```python
from build123d import *

# Parameters (mm, degrees)
F1_DEPTH  = 6.35
F2_W      = 7.9056663411
F2_H      = 7.9056663411
F3_DEPTH  = 25.4
F4_W      = 6.858
F4_H      = 6.858
F5_DEPTH  = 25.4
F6_W      = 7.9056663411
F6_H      = 8.1499283314
F6_W_2    = 8.1499283314
F6_H_2    = 7.9056663411
F7_DEPTH  = 1.27
F8_SIZE   = 1.26999
F10_DEPTH = 6.35


# Not quite as in the source:
# - a fillet or chamfer is up to 0.001 mm smaller than in the source, because OpenCascade refuses the exact size
# - a feature names something its author has since deleted; it is built from what else it names


with BuildPart() as f1:
    # F0 (on Top) → F1 (new body)
    with BuildSketch(Plane.XY):
        with BuildLine():
            ThreePointArc((13.6716806904, 59.1812469065), (-3.4947036843, 66.2917961397), (3.6158455206, 49.1254117533))
            ThreePointArc((3.6158455206, 49.1254117533), (10.7263947587, 52.0706976733), (13.6716806904, 59.1812469065))
        make_face()
    extrude(amount=F1_DEPTH)

    # F4 (on face) → F5 (cut)
    with BuildSketch(Plane.XY.offset(6.35)):
        with Locations((3.6158455372, 59.1812469065)):
            Rectangle(F4_W, F4_H)
    extrude(amount=-F5_DEPTH, mode=Mode.SUBTRACT)



with BuildPart() as f1b:
    # F0 (on Top) → F1, piece 2 (new body)
    with BuildSketch(Plane.XY):
        Polygon((3.6158455206, 49.1254117533), (-34.4841544628, 49.1254117533), (-34.4841544628, -27.0745882467), (41.7158455372, -27.0745882467), (41.7158455372, 49.1254117533), align=None)
    extrude(amount=F1_DEPTH)

    # F2 (on face) → F3 (cut)
    with BuildSketch(Plane.XY.offset(6.35)):
        Polygon((-34.4841544628, 33.0698170808), (-26.3342261314, 33.0698170808), (-18.4285597903, 33.0698170808), (-18.4285597903, 40.9754834219), (-18.4285597903, 49.1254117533), (-34.4841544628, 49.1254117533), align=None)
        Polygon((25.6602508647, 40.9754834219), (25.6602508647, 33.0698170808), (33.5659172058, 33.0698170808), (41.7158455372, 33.0698170808), (41.7158455372, 49.1254117533), (25.6602508647, 49.1254117533), align=None)
        Polygon((33.5659172058, -11.0189935742), (25.6602508647, -11.0189935742), (25.6602508647, -18.9246599153), (25.6602508647, -27.0745882467), (41.7158455372, -27.0745882467), (41.7158455372, -11.0189935742), align=None)
        Polygon((-18.4285597903, -18.9246599153), (-18.4285597903, -11.0189935742), (-26.3342261314, -11.0189935742), (-34.4841544628, -11.0189935742), (-34.4841544628, -27.0745882467), (-18.4285597903, -27.0745882467), align=None)
        with Locations((-22.3813929609, 1.0837679277)):
            Rectangle(F2_W, F2_H)
        with Locations((-22.3813929609, 20.9670555789)):
            Rectangle(F2_W, F2_H)
        with Locations((-6.3257982884, 37.0226502514)):
            Rectangle(F2_W, F2_H)
        with Locations((-6.3257982884, 20.9670555789)):
            Rectangle(F2_W, F2_H)
        with Locations((-6.3257982884, 1.0837679277)):
            Rectangle(F2_W, F2_H)
        with Locations((-6.3257982884, -14.9718267448)):
            Rectangle(F2_W, F2_H)
        with Locations((13.5574893628, -14.9718267448)):
            Rectangle(F2_W, F2_H)
        with Locations((13.5574893628, 1.0837679277)):
            Rectangle(F2_W, F2_H)
        with Locations((29.6130840353, 1.0837679277)):
            Rectangle(F2_W, F2_H)
        with Locations((29.6130840353, 20.9670555789)):
            Rectangle(F2_W, F2_H)
        with Locations((13.5574893628, 20.9670555789)):
            Rectangle(F2_W, F2_H)
        with Locations((13.5574893628, 37.0226502514)):
            Rectangle(F2_W, F2_H)
    extrude(amount=-F3_DEPTH, mode=Mode.SUBTRACT)

    # F6 (on face) → F7 (join, symmetric)
    with BuildSketch(Plane.XY.offset(6.35)):
        with Locations((-22.3813929609, 28.9948529151)):
            Rectangle(F6_W, F6_H)
        with Locations((-14.3535956246, 28.9948529151)):
            Rectangle(F6_W_2, F6_H)
        with Locations((-14.3535956246, 37.0226502514)):
            Rectangle(F6_W_2, F6_H_2)
        with Locations((-6.3257982884, 28.9948529151)):
            Rectangle(F6_W, F6_H)
        with Locations((-14.3535956246, 20.9670555789)):
            Rectangle(F6_W_2, F6_H_2)
        with Locations((13.5574893628, 28.9948529151)):
            Rectangle(F6_W, F6_H)
        with Locations((29.6130840353, 28.9948529151)):
            Rectangle(F6_W, F6_H)
        with Locations((21.585286699, 28.9948529151)):
            Rectangle(F6_W_2, F6_H)
        with Locations((21.585286699, 37.0226502514)):
            Rectangle(F6_W_2, F6_H_2)
        with Locations((21.585286699, 20.9670555789)):
            Rectangle(F6_W_2, F6_H_2)
        with Locations((-14.3535956246, 1.0837679277)):
            Rectangle(F6_W_2, F6_H_2)
        with Locations((-14.3535956246, -6.9440294085)):
            Rectangle(F6_W_2, F6_H)
        with Locations((-14.3535956246, -14.9718267448)):
            Rectangle(F6_W_2, F6_H_2)
        with Locations((-22.3813929609, -6.9440294085)):
            Rectangle(F6_W, F6_H)
        with Locations((-6.3257982884, -6.9440294085)):
            Rectangle(F6_W, F6_H)
        with Locations((13.5574893628, -6.9440294085)):
            Rectangle(F6_W, F6_H)
        with Locations((21.585286699, -6.9440294085)):
            Rectangle(F6_W_2, F6_H)
        with Locations((29.6130840353, -6.9440294085)):
            Rectangle(F6_W, F6_H)
        with Locations((21.585286699, -14.9718267448)):
            Rectangle(F6_W_2, F6_H_2)
        with Locations((21.585286699, 1.0837679277)):
            Rectangle(F6_W_2, F6_H_2)
    extrude(amount=F7_DEPTH, both=True)

    # F8 (size 1.27 in the source; OpenCascade refuses exactly that, so slightly less here)
    f8_edges = [f1b.edges().sort_by_distance(p)[0] for p in [
        (-22.381393, 33.069817, 7.62),
        (-18.42856, 37.02265, 7.62),
        (-14.353596, 40.975483, 7.62),
        (-10.278631, 37.02265, 7.62),
        (-6.325798, 33.069817, 7.62),
        (-2.372965, 28.994853, 7.62),
        (-6.325798, 24.919889, 7.62),
        (-10.278631, 20.967056, 7.62),
        (-14.353596, 17.014222, 7.62),
        (-18.42856, 20.967056, 7.62),
        (-22.381393, 24.919889, 7.62),
        (-26.334226, 28.994853, 7.62),
        (-10.278631, 1.083768, 7.62),
        (-6.325798, -2.869065, 7.62),
        (-2.372965, -6.944029, 7.62),
        (-6.325798, -11.018994, 7.62),
        (-14.353596, -18.92466, 7.62),
        (-26.334226, -6.944029, 7.62),
        (-22.381393, -11.018994, 7.62),
        (-18.42856, -14.971827, 7.62),
        (-22.381393, -2.869065, 7.62),
        (-18.42856, 1.083768, 7.62),
        (-14.353596, 5.036601, 7.62),
        (-10.278631, -14.971827, 7.62),
        (25.660251, 1.083768, 7.62),
        (25.660251, -14.971827, 7.62),
        (21.585287, -18.92466, 7.62),
        (17.510323, -14.971827, 7.62),
        (13.557489, -11.018994, 7.62),
        (9.604656, -6.944029, 7.62),
        (13.557489, -2.869065, 7.62),
        (17.510323, 1.083768, 7.62),
        (21.585287, 5.036601, 7.62),
        (29.613084, -2.869065, 7.62),
        (29.613084, -11.018994, 7.62),
        (33.565917, -6.944029, 7.62),
        (29.613084, 33.069817, 7.62),
        (25.660251, 37.02265, 7.62),
        (21.585287, 40.975483, 7.62),
        (17.510323, 37.02265, 7.62),
        (13.557489, 33.069817, 7.62),
        (9.604656, 28.994853, 7.62),
        (17.510323, 20.967056, 7.62),
        (13.557489, 24.919889, 7.62),
        (21.585287, 17.014222, 7.62),
        (29.613084, 24.919889, 7.62),
        (33.565917, 28.994853, 7.62),
        (25.660251, 20.967056, 7.62),
    ]]
    chamfer(f8_edges, length=F8_SIZE)


with BuildPart() as f1_1:
    add(f1.part)

    add(f1b.part)  # F10 merges F1b
    # F9 (on face) → F10 (join)
    with BuildSketch(Plane.XY.offset(6.35)):
        with BuildLine():
            Line((-6.439989616, 49.1254117533), (3.6158455372, 49.1254117533))
            ThreePointArc((3.6158455372, 49.1254117533), (-3.4947036902, 52.0706976792), (-6.439989616, 59.1812469065))
            Line((-6.439989616, 59.1812469065), (-6.439989616, 49.1254117533))
        make_face()
        with BuildLine():
            Line((3.6158455372, 49.1254117533), (13.6716806904, 49.1254117533))
            Line((13.6716806904, 49.1254117533), (13.6716806904, 59.1812469065))
            ThreePointArc((13.6716806904, 59.1812469065), (10.7263947645, 52.0706976792), (3.6158455372, 49.1254117533))
        make_face()
    extrude(amount=-F10_DEPTH)


solid = f1_1.part
```
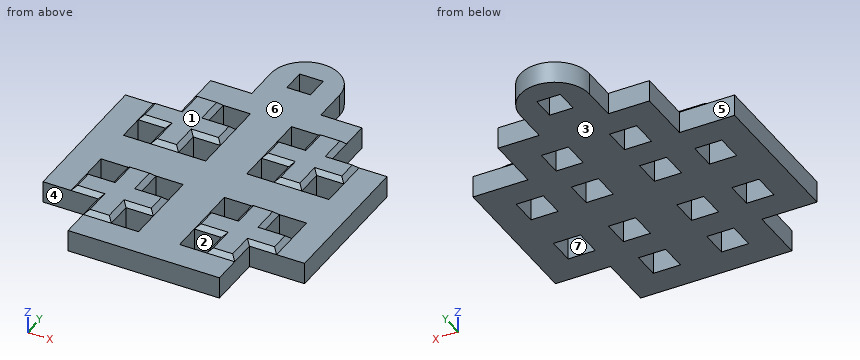
For this review, take the finished solid that the model builds, in its own axes (mm). Face numbers are marked on the shaded views. A direction names the side the tool comes from. Coordinates: 2 decimals unless noted, no trailing zeros. Order: outer loops, then holes, each group sorted by start corner. A loop starts at its lowest first (then second) coordinate and runs counter-clockwise, first axis right, second up. Notation, with made-up numbers: (29.5, 58) -> (74.5, 58) arc R17 ccw to (74.5, 89) -> close; hole circle Ø6 at (66.25, -37.5). An arc over 180 degrees is marked (long way). Use CSV: the item, a comma, the result in double quotes. Start each with the question number.
Item 1: Draft analysis for pull direction X (two halves, no side actions). For the marked faces 1 and 2, state which applies: pulls with the +X half, pulls with the -X half, needs draft (parallel to the pull), parting line crosses it, or undercut.
Item 2: Wall thickness on probe 1 along X at (y, z) = (3, 3.75); probe 2 along Y at (x, z) = (-21.5, 4.5); probe 3 along Y at (x, z) = (-30.5, 6): over which ranges is each line inside the solid? List them lowest first.
Item 3: We need section B-B, the plane y = 1.5. Give the boundary of the cut face in (x, z).
Item 4: We need section A-A, the plane x = 29. Give the boundary of the cut face in (y, z).
Item 5: Insertion check: pin 1 (3 mm diameter, centred on x = -22.5, z = 4, fed in from +Y); pin 2 (1.5 mm diameter, centred on x = -1.5, z = 5, fed in from +Y); pin 3 (3 mm diameter, centred on y = -14.5, z = 2.5, fed in from -X). Each pin has a flat end and moves straight along its axis. Give the tip position at first contact, or say it passes through.
Item 6: For the marked faces 3, 4, 5, 6 and 7, list the 3-axis set-ups (+Z, -Z, +X, -X, +Y, -Y) from which the entire face can be reached by the end or side of a thin tool; tool diameter is ignored.
Derived:
1,face 1,"needs draft"
1,face 2,"undercut"
2,probe 1,"x = -34.48 to -26.33, -18.43 to -10.28, -2.37 to 9.6, 17.51 to 25.66, 33.57 to 41.72"
2,probe 2,"y = -11.02 to -2.87, 5.04 to 17.01, 24.92 to 33.07"
2,probe 3,"y = -11.02 to 33.07"
3,outline,"(-34.48, 0) -> (-26.33, 0) -> (-26.33, 6.35) -> (-34.48, 6.35) -> close; (-18.43, 0) -> (-10.28, 0) -> (-10.28, 6.35) -> (-11.55, 7.62) -> (-17.16, 7.62) -> (-18.43, 6.35) -> close; (-2.37, 0) -> (9.6, 0) -> (9.6, 6.35) -> (-2.37, 6.35) -> close; (17.51, 0) -> (25.66, 0) -> (25.66, 6.35) -> (24.39, 7.62) -> (18.78, 7.62) -> (17.51, 6.35) -> close; (33.57, 0) -> (41.72, 0) -> (41.72, 6.35) -> (33.57, 6.35) -> close"
4,outline,"(-11.02, 0) -> (-2.87, 0) -> (-2.87, 6.35) -> (-4.14, 7.62) -> (-9.75, 7.62) -> (-11.02, 6.35) -> close; (5.04, 0) -> (17.01, 0) -> (17.01, 6.35) -> (5.04, 6.35) -> close; (24.92, 0) -> (33.07, 0) -> (33.07, 6.35) -> (31.8, 7.62) -> (26.19, 7.62) -> (24.92, 6.35) -> close"
5,pin 1,"stops at y = 33.07"
5,pin 2,"stops at y = 68.24"
5,pin 3,"stops at x = -18.43"
6,face 3,"-Z, +X, -X, +Y, -Y"
6,face 4,"+Z, -Z, -X, -Y"
6,face 5,"+Z, -Z, -X, +Y"
6,face 6,"+Z"
6,face 7,"+Z, -Z"
